Input: dimensioned drawing with shaded views. Units: mm. Origin: part minimum x, y, z. A direction names the side the tool comes from. Round coordinates to 2 decimals unless told otherwise and drop trailing zeros. Loops run counter-clockwise (first coordinate to the right, second up) from the corner with the lowest first, then second, coordinate; pieces in that order, holes last. Notation, with made-up numbers: (54.25, 69) - (87.25, 69) arc R23 cw to (87.25, 96) - close; hole circle Ø1 at (37, 46). An arc over 180 degrees is marked (long way). Write each question's results on one line, items separated by ' | '.
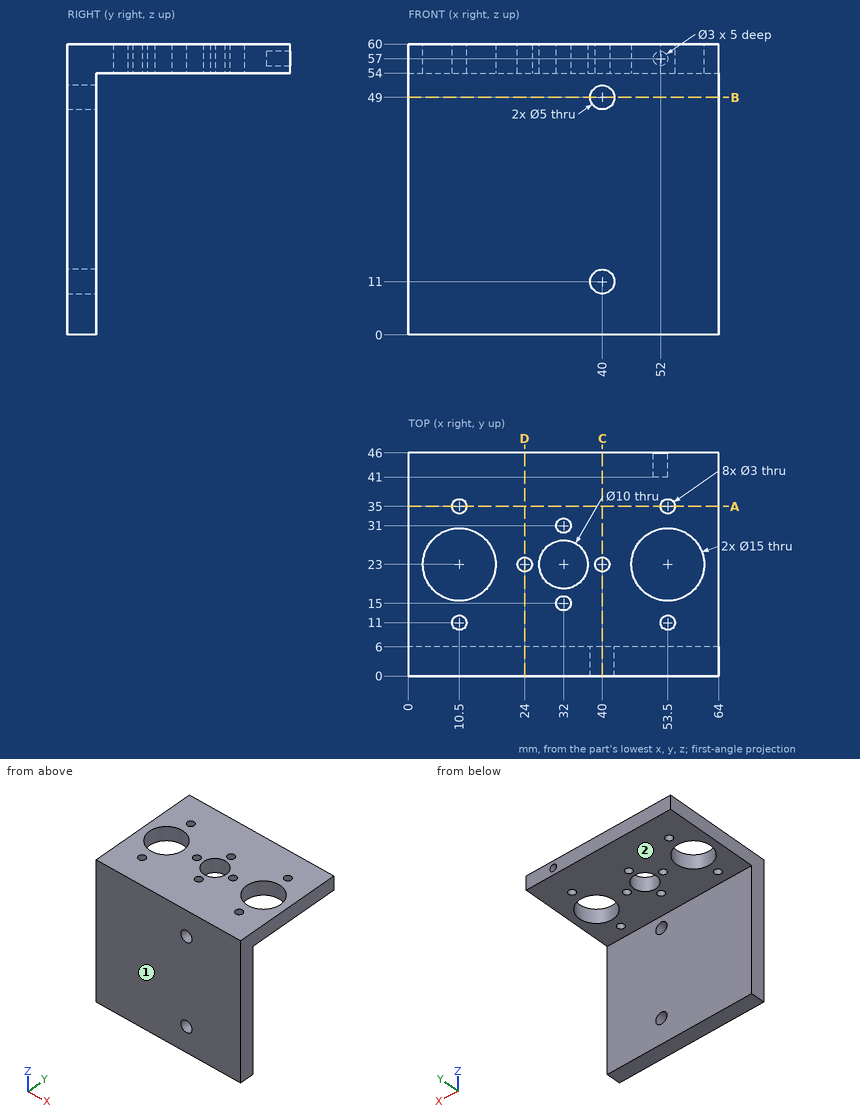
1. Set-up query: the marked faces 1 and 2. Return all of +Z, -Z, +X, -X, +Y, -Y with unobstructed straight access to the full face (end or side cutting, diameter ignored); none if empty.
Answer:
face 1: +Z, -Z, +X, -X, -Y | face 2: -Z, +X, -X, +Y
2. Section query D-D, the plane x = 24. Output: boundary loops of the cut face in (y, z), plus the area to 3 significant figures.
Answer:
outline: (0, 0) - (6, 0) - (6, 54) - (21.5, 54) - (21.5, 60) - (0, 60) - close; (24.5, 54) - (46, 54) - (46, 60) - (24.5, 60) - close | area: 582 mm^2
3. Line query: line 1 (Y direction, x = 10.5, z = 55.4); line 2 (Z direction, x = 32, y = 33); line 3 (Y direction, x = 43, z = 20.5). Output: solid intervals per line, ascending. Write a range as [from, to].
Answer:
line 1: [0, 9.5], [12.5, 15.5], [30.5, 33.5], [36.5, 46] | line 2: [54, 60] | line 3: [0, 6]
4. Section query C-C, the plane x = 40. Output: boundary loops of the cut face in (y, z), plus the area to 3 significant figures.
Answer:
outline: (0, 0) - (6, 0) - (6, 8.5) - (0, 8.5) - close; (0, 13.5) - (6, 13.5) - (6, 46.5) - (0, 46.5) - close; (0, 51.5) - (6, 51.5) - (6, 54) - (21.5, 54) - (21.5, 60) - (0, 60) - close; (24.5, 54) - (46, 54) - (46, 60) - (24.5, 60) - close | area: 522 mm^2
5. Section query B-B, the plane z = 49. Output: boundary loops of the cut face in (x, y).
Answer:
outline: (0, 0) - (37.5, 0) - (37.5, 6) - (0, 6) - close; (42.5, 0) - (64, 0) - (64, 6) - (42.5, 6) - close
6. Section query A-A, the plane y = 35. Output: boundary loops of the cut face in (x, z).
Answer:
outline: (0, 54) - (9, 54) - (9, 60) - (0, 60) - close; (12, 54) - (52, 54) - (52, 60) - (12, 60) - close; (55, 54) - (64, 54) - (64, 60) - (55, 60) - close
7. Contact query for flat-ended pins moving along their axis: pin 1 (10 mm diameter, centred on x = 28.5, y = 36, fed in from -Z); pin 2 (3 mm diameter, centred on x = 29, z = 44, fed in from +Y); pin 3 (1.8 mm diameter, centred on x = 52, z = 57, fed in from +Y). Output: stop coordinate, or through.
Answer:
pin 1: z = 54 | pin 2: y = 6 | pin 3: y = 41
